Geometry check sheet. Reference: the model listing, model coordinates, mm. A direction names the side the tool comes from. Round coordinates to 2 decimals unless told otherwise and drop trailing zeros. Order: outer loops, then holes, each group sorted by start corner. A loop starts at its lowest first (then second) coordinate and runs counter-clockwise, first axis right, second up.
(1) Set-up check for faces 5 (the face through (3.874, 11.458, 0.86)), 6 (the face through (-5, 25.4, 0)), 7 (the face through (-3, 21.431, 1)): record each of +Z, -Z, +X, -X, +Y, -Y from which the full face is reachable in a straight line by a thin tool's end or side.
(2) Sectioned sample at A-A (y = 13.5). Record the boundary of the cut face in (x, z).
(3) Go/stop test with flat-tipped pins: pin 1 (3 mm diameter, centred on y = 13.5, z = -0.5, fed in from +X); pin 2 (4 mm diameter, centred on x = -0.5, y = 34, fed in from +Z); pin 3 (4 mm diameter, centred on x = 4.5, y = 30.5, fed in from +Z); pin 4 (0.8 mm diameter, centred on x = -5.5, z = -2, fed in from +Y). Record where each tip stops, or that it passes through.
(4) Release check for a two-part mould opening along Y. For faces 1 (the face through (2.984, 32, 0)), 2 (the face through (-1, 23.812, -3)), 3 (the face through (0, 0, 0)), 4 (the face through (5, 25.4, 0)) record: +Y half, -Y half, draft (parallel to the pull), parting line (faces both ways), or undercut.
(5) Material ranges on line 1 along X through (y, z) = (33, 0.75); line 2 along Y through (x, z) = (-5, -1.5); line 3 along Y through (x, z) = (-3.5, 0), recorded low to high.
from build123d import *

# Parameters (mm, degrees)
CUT_EXTRUDE1_DEPTH      = 40.103215572
CUT_EXTRUDE1_DEPTH_BACK = 40.103215572
CHAMFER1_SIZE           = 1.016
CHAMFER1_SIZE2          = 1.75976362
FILLET1_R               = 0.79375


with BuildPart() as part:
    # Sketch1 → Revolve1 (revolve)
    with BuildSketch(Plane.XY, mode=Mode.PRIVATE) as revolve1_sk:
        with BuildLine():
            Line((6.223, 36.649006265), (6.223, 23.8125))
            Line((6.223, 23.8125), (2.9845, 23.8125))
            Line((2.9845, 23.8125), (2.9845, 21.43125))
            Line((2.9845, 21.43125), (3.96875, 21.43125))
            Line((3.96875, 21.43125), (3.96875, 0))
            Line((3.96875, 0), (0, 0))
            Line((0, 0), (0, 38.1))
            ThreePointArc((0, 38.1), (3.175227984, 37.647818746), (6.223, 36.649006265))
        make_face()
    revolve(revolve1_sk.sketch.rotate(Axis((0, 0, 0), (0, 1, 0)), 90), axis=Axis((0, 0, 0), (0, 1, 0)))

    # Sketch2 → Cut-Extrude1 (cut, two sides: drawn at the far end of the back side and taken through both)
    with BuildSketch(Plane.XY.offset(-CUT_EXTRUDE1_DEPTH_BACK)):
        with BuildLine():
            Line((-6.223, 25.4), (-4.572, 25.4))
            ThreePointArc((-4.572, 25.4), (-3.449467985, 25.864967985), (-2.9845, 26.9875))
            Line((-2.9845, 26.9875), (-2.9845, 38.1))
            Line((-2.9845, 38.1), (-6.223, 38.1))
            Line((-6.223, 38.1), (-6.223, 25.4))
        make_face()
        with BuildLine():
            Line((6.223, 38.1), (6.223, 25.4))
            Line((6.223, 25.4), (4.572, 25.4))
            ThreePointArc((4.572, 25.4), (3.449467985, 25.864967985), (2.9845, 26.9875))
            Line((2.9845, 26.9875), (2.9845, 38.1))
            Line((2.9845, 38.1), (6.223, 38.1))
        make_face()
    extrude(amount=CUT_EXTRUDE1_DEPTH + CUT_EXTRUDE1_DEPTH_BACK, mode=Mode.SUBTRACT)

    # Chamfer1
    chamfer1_edges = [part.edges().sort_by_distance(p)[0] for p in [
        (0, 0, 3.96875),
    ]]
    chamfer1_side = [part.faces().sort_by_distance(p)[0] for p in [
        (0, 0, 0),
    ]]
    chamfer(chamfer1_edges, length=CHAMFER1_SIZE, length2=CHAMFER1_SIZE2, reference=chamfer1_side[0])

    # Fillet1
    fillet1_edges = [part.edges().sort_by_distance(p)[0] for p in [
        (1.540166147, 36.649006265, -6.029396092),
        (0, 36.649006265, 6.223),
    ]]
    fillet(fillet1_edges, radius=FILLET1_R)


solid = part.part
Answer below:
1. face 5: -Y
1. face 6: +Z, -Z, -X, +Y
1. face 7: none
2. outline: circle Ø7.94 at (0, 0)
3. pin 1: stops at x = 3.97
3. pin 2: stops at z = 6.22
3. pin 3: stops at z = 5.7
3. pin 4: stops at y = 25.4
4. face 1: draft
4. face 2: undercut
4. face 3: -Y half
4. face 4: +Y half
5. line 1: x = -2.98 to 2.98
5. line 2: y = 23.81 to 25.4
5. line 3: y = 0.95 to 21.43, 23.81 to 25.82
